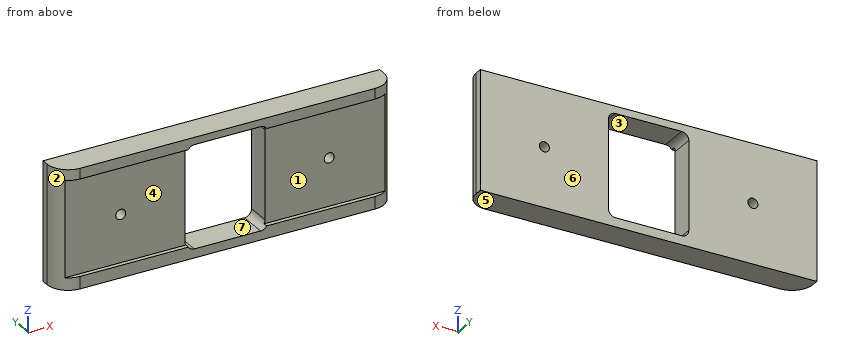
from build123d import *

# Parameters (mm, degrees)
SKETCH1_W               = 76.2
SKETCH1_H               = 26.809375
BOSS_EXTRUDE1_DEPTH     = 6.35
FILLET1_R               = 4.7625
SKETCH2_W               = 21.65
SKETCH2_H               = 1
CUT_EXTRUDE1_DEPTH      = 80.112608871
CUT_EXTRUDE2_DEPTH      = 63.558479955
CUT_EXTRUDE2_DEPTH_BACK = 63.558479955
F_4_40_TAPPED_HOLE1_D   = 2.2606


with BuildPart() as part:
    # Sketch1 → Boss-Extrude1 (new body)
    with BuildSketch(Plane(origin=(0, 0, 0), x_dir=(1, 0, 0), z_dir=(0, 1, 0))):
        with Locations((-20.831303498, 6.894139619)):
            Rectangle(SKETCH1_W, SKETCH1_H)
    extrude(amount=BOSS_EXTRUDE1_DEPTH)

    # Fillet1
    fillet1_edges = [part.edges().sort_by_distance(p)[0] for p in [
        (-58.931303498, 0, -6.894139619),
        (17.268696502, 0, -6.894139619),
    ]]
    fillet(fillet1_edges, radius=FILLET1_R)

    # Sketch2 → Cut-Extrude1 (cut, through all)
    with BuildSketch(Plane(origin=(17.268696502, 0, 0), x_dir=(0, 0, -1), z_dir=(1, 0, 0))):
        with Locations((6.695702119, 0.5)):
            Rectangle(SKETCH2_W, SKETCH2_H)
    extrude(amount=-CUT_EXTRUDE1_DEPTH, mode=Mode.SUBTRACT)

    # Sketch3 → Cut-Extrude2 (cut, two sides: drawn at the far end of the back side and taken through both)
    with BuildSketch(Plane.XZ.offset(-1).offset(-CUT_EXTRUDE2_DEPTH_BACK)):
        with BuildLine():
            Line((-11.743803498, 3.304297881), (-11.743803498, -16.695702119))
            ThreePointArc((-11.743803498, -16.695702119), (-12.208771483, -17.818234134), (-13.331303498, -18.283202119))
            Line((-13.331303498, -18.283202119), (-28.331303498, -18.283202119))
            ThreePointArc((-28.331303498, -18.283202119), (-29.453835513, -17.818234134), (-29.918803498, -16.695702119))
            Line((-29.918803498, -16.695702119), (-29.918803498, 3.304297881))
            ThreePointArc((-29.918803498, 3.304297881), (-29.453835513, 4.426829896), (-28.331303498, 4.891797881))
            Line((-28.331303498, 4.891797881), (-13.331303498, 4.891797881))
            ThreePointArc((-13.331303498, 4.891797881), (-12.208771483, 4.426829896), (-11.743803498, 3.304297881))
        make_face()
    extrude(amount=CUT_EXTRUDE2_DEPTH + CUT_EXTRUDE2_DEPTH_BACK, mode=Mode.SUBTRACT)

    # #4-40 Tapped Hole1 (through all)
    with Locations(Plane(origin=(0, 6.35, 0), x_dir=(-1, 0, 0), z_dir=(0, 1, 0))):
        with Locations((44.425053498, -6.794920869), (-2.762446502, -6.794920869)):
            Hole(F_4_40_TAPPED_HOLE1_D / 2)


solid = part.part
Input: part model. Units: mm. Frame: model coordinates. Face numbers are marked on the shaded views. A direction names the side the tool comes from. Coordinates: 2 decimals unless noted, no trailing zeros. Loops run counter-clockwise (first coordinate to the right, second up) from the corner with the lowest first, then second, coordinate; pieces in that order, holes last. Notation, with made-up numbers: (2, 84.25) - (43, 84.25) arc R30 ccw to (43, 108.25) - close; hole circle Ø1 at (-13, 29). An arc over 180 degrees is marked (long way). Answer in a Markdown table with one row per item. Add a question column.
Item 1: Access query for the marked faces 1, 2 and 3. Directions: +Z, -Z, +X, -X, +Y, -Y. A direction counts if a zero-diameter tool reaches every point of the face in a straight line with its end or side. Return the directions, or none.
Item 2: Section query B-B on x = 9.5. Return the cut outline in (y, z), then the cut area to 3 significant figures.
Item 3: Mould query, pull axis Z, two halves, no side actions, for the marked faces 4, 5, 6 and 7. Classes: released by +Z, released by -Z, zero draft, split by the parting line, or undercut.
Item 4: Section query D-D on y = 5.5. Return the cut outline in (x, z) (1 decimal), then the cut area to 3 significant figures.
Item 5: Contact query for flat-ended pins moving along their axis: P1, Ø1, axis at y = 1, z = -2.5, coming from the -X side; P2, Ø1.6, axis at y = 3.5, z = -5.5, coming from the -X side; P3, Ø1, axis at y = 4, z = -15, coming from the +X side. Output: stop coordinate, or through.
Item 6: Section query C-C on y = 1.75. Return the cut outline in (x, z) (1 decimal).
Item 7: Line query: line 1 along Z through (x, y) = (-27.5, 2); line 2 along Z through (x, y) = (-11, 0.5); line 3 along X through (y, z) = (5.5, -13.25). Output: solid intervals per line, ascending. Write a range as [from, to].
Recorded:
| question | item | result |
|---|---|---|
| 1 | face 1 | +X, -X, -Y |
| 1 | face 2 | +Z, -Z, -X, -Y |
| 1 | face 3 | +Y, -Y |
| 2 | outline | (0, -20.3) - (6.35, -20.3) - (6.35, 6.51) - (0, 6.51) - (0, 4.13) - (1, 4.13) - (1, -17.52) - (0, -17.52) - close |
| 2 | area | 149 mm^2 |
| 3 | face 4 | undercut |
| 3 | face 5 | released by -Z |
| 3 | face 6 | zero draft |
| 3 | face 7 | undercut |
| 4 | outline | (-58.9, -20.3) - (17.3, -20.3) - (17.3, 6.5) - (-58.9, 6.5) - close; hole circle Ø2.3 at (-44.4, -6.8); hole (-29.9, -16.7) arc R1.6 ccw to (-28.3, -18.3) - (-13.3, -18.3) arc R1.6 ccw to (-11.7, -16.7) - (-11.7, 3.3) arc R1.6 ccw to (-13.3, 4.9) - (-28.3, 4.9) arc R1.6 ccw to (-29.9, 3.3) - close; hole circle Ø2.3 at (2.8, -6.8) |
| 4 | area | 1,620 mm^2 |
| 5 | P1 | x = -57.64 |
| 5 | P2 | x = -58.91 |
| 5 | P3 | x = 17.26 |
| 6 | outline | (-57.9, -20.3) - (16.2, -20.3) - (16.2, 6.5) - (-57.9, 6.5) - close; hole circle Ø2.3 at (-44.4, -6.8); hole (-29.9, -16.7) arc R1.6 ccw to (-28.3, -18.3) - (-13.3, -18.3) arc R1.6 ccw to (-11.7, -16.7) - (-11.7, 3.3) arc R1.6 ccw to (-13.3, 4.9) - (-28.3, 4.9) arc R1.6 ccw to (-29.9, 3.3) - close; hole circle Ø2.3 at (2.8, -6.8) |
| 7 | line 1 | [-20.3, -18.28], [4.89, 6.51] |
| 7 | line 2 | [-20.3, -17.52], [4.13, 6.51] |
| 7 | line 3 | [-58.93, -29.92], [-11.74, 17.27] |
